from build123d import *

# Parameters (mm, degrees)
SWEEP_START         = 9.9999999
SWEEP_1_OUTLINE_R   = 5
SWEEP_1_DEPTH       = 15.0000001
SWEEP_START_2       = -25
SWEEP_1_2_OUTLINE_R = 5
SWEEP_1_2_DEPTH     = 15
SWEEP_1_3_OUTLINE_R = 5
SWEEP_1_3_ANGLE     = 90
SKETCH_2_R          = 3.924596356


with BuildPart() as part:
    # Sweep 1: read off the stored shape, not the designer's step
    # Sweep 1 outline → Sweep 1 (new body)
    with BuildSketch(Plane(origin=(0, 0, 0), x_dir=(1, 0, 0), z_dir=(0, 1, 0)).offset(SWEEP_START)):
        Circle(SWEEP_1_OUTLINE_R)
    extrude(amount=SWEEP_1_DEPTH)



with BuildPart() as body_2:
    # Sweep 1 2 outline → Sweep 1 2 (new body)
    with BuildSketch(Plane.YZ.offset(SWEEP_START_2)):
        Circle(SWEEP_1_2_OUTLINE_R)
    extrude(amount=SWEEP_1_2_DEPTH)


with BuildPart() as part_1:
    add(part.part)

    add(body_2.part)  # Sweep 1 3 merges body 2
    # Sweep 1 3 outline → Sweep 1 3 (revolve)
    with BuildSketch(Plane(origin=(-10, 10, 0), x_dir=(0, -1, 0), z_dir=(-1, 0, 0))):
        with Locations((10, 0)):
            Circle(SWEEP_1_3_OUTLINE_R)
    revolve(axis=Axis((-10, 10, 0), (0, 0, 1)), revolution_arc=SWEEP_1_3_ANGLE)

    # Sweep 1 4: sweep along a path in 草图4
    with BuildLine(Plane.XY) as sweep_1_4_path:
        Line((0, 25.105232373), (0, 10))
        ThreePointArc((0, 10), (-2.928932188, 2.928932188), (-10, 0))
        Line((-10, 0), (-25, 0))
    # 草图2 → Sweep 1 4 (sweep, cut)
    with BuildSketch(Plane.ZY.offset(25)):
        Circle(SKETCH_2_R)
    sweep(path=sweep_1_4_path.line, mode=Mode.SUBTRACT)


solid = part_1.part
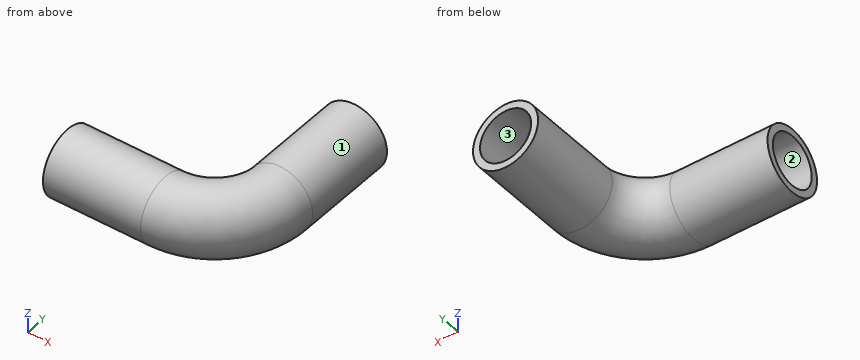
CAD build for the part. Positions are in the model's coordinates, mm. Face numbers are marked on the shaded views. Round coordinates to 2 decimals unless told otherwise and drop trailing zeros. Order: outer loops, then holes, each group sorted by start corner. A loop starts at its lowest first (then second) coordinate and runs counter-clockwise, first axis right, second up. Notation, with made-up numbers: (3.25, -11) -> (51.25, -11) arc R20 cw to (51.25, -4) -> close; hole circle Ø4 at (13, 56.25). An arc over 180 degrees is marked (long way). Write item = value, one per line. Start each with the question number.
(1) Pull direction X, two halves, no side cores. Call the marked faces 1, 2 and 3: released by +X, released by -X, zero draft, split by the parting line, or undercut.
(2) Probe line 1 (Z direction, x = 0, y = 21.5). List the from-to ranges inside material, lowest first. Write a range as [from, to].
(3) Cut at B-B, the plane x = -20.5. List the corners of the cut face in (y, z).
(4) Pin check, flat tips, straight feed: P1, Ø1.5, axis at x = -19, y = 3.5, coming from the +Z side; P2, Ø5, axis at x = -5, z = -1.5, coming from the -Y side; P3, Ø1, axis at x = -19.5, z = 3, coming from the +Y side. Stop position of each tip, or through.
(5) Cut at A-A, the plane z = 0. List the corners of the cut face in (x, y), then the cut area to 3 significant figures.
Model answer:
q1.face_1 = split by the parting line
q1.face_2 = zero draft
q1.face_3 = undercut
q2.line_1 = [-5, -3.92], [3.92, 5]
q3.outline = circle Ø10 at (0, 0); hole circle Ø7.85 at (0, 0)
q4.P1 = 4.18
q4.P2 = -4.73
q4.P3 = 4.33
q5.outline = (-25, -5) -> (-10, -5) arc R15 ccw to (5, 10) -> (5, 25) -> (3.92, 25) -> (3.92, 10) arc R13.92 cw to (-10, -3.92) -> (-25, -3.92) -> close; (-25, 3.92) -> (-10, 3.92) arc R6.08 ccw to (-3.92, 10) -> (-3.92, 25) -> (-5, 25) -> (-5, 10) arc R5 cw to (-10, 5) -> (-25, 5) -> close
q5.area = 98.3 mm2
